Here's how the part is built. I have some questions about the finished solid (model axes, mm). Give positions to 0.01 mm unless a question says otherwise; leave off trailing zeros. Order: outer loops, then holes, each group sorted by start corner. A loop starts at its lowest first (then second) coordinate and runs counter-clockwise, first axis right, second up. Notation, with made-up numbers: (51, -31) -> (107, -31) arc R7 ccw to (107, -25) -> close; hole circle Ø4 at (-39.5, -5). An arc over 180 degrees is marked (long way). Write each question's results on one line, items separated by ' | '. Start each with the question number.
Q1. Imagine slicing it at A-A, the plane z = 4.25. Please give me the cut outline in (x, y).
Q2. Thinking about a two-plate mould opening in X: for faces 1 (the face through (-0.816, -34.994, 3.944)), 2 (the face through (0, -40, 10)), 3 (the face through (-1.24, -30.58, 4.93)), which applies, pulls with the +X half, pulls with the -X half, needs draft (parallel to the pull), parting line crosses it, or undercut?
Q3. Imagine slicing it at C-C, the plane z = 8.5. Please give me the cut outline in (x, y), then the cut area to 3 significant figures.
Q4. I'm going to push flat-ended pins straight in: pin 1 (3 mm diameter, centred on x = -5.12, y = -43.58, fed in from +Z); pin 2 (3 mm diameter, centred on y = -32.5, z = 6, fed in from +X); pin 3 (3 mm diameter, centred on x = 5.66, y = -42.64, fed in from -Z); pin 4 (3 mm diameter, centred on y = -34.5, z = 4, fed in from -X). Where does each tip first touch, or does it pass through?
Q5. Imagine slicing it at B-B, the plane x = -5.25. State how many separate pieces and enclosed holes the cut face has, then the cut area to 3 significant figures.
Q6. I need wall thicknesses on line 1 along Y through (x, z) = (1.5, 9.25); line 2 along Y through (x, z) = (5.5, 9.5); line 3 along Y through (x, z) = (1, 5). Which ranges of each line are inside material? Lowest first, please. Write a range as [from, to].
```python
from build123d import *

# Parameters (mm, degrees)
SKETCH1_R           = 9.5
SKETCH1_R_2         = 1.25
BOSS_EXTRUDE1_DEPTH = 10
CHAMFER1_SIZE       = 2
CHAMFER2_SIZE       = 2


with BuildPart() as part:
    # Sketch1 → Boss-Extrude1 (new body)
    with BuildSketch(Plane.XY):
        with Locations((0, -40)):
            Circle(SKETCH1_R)
        with Locations((5.119700277, -36.415147273)):
            Circle(SKETCH1_R_2, mode=Mode.SUBTRACT)
        with Locations((0.544723392, -46.226216863)):
            Circle(SKETCH1_R_2, mode=Mode.SUBTRACT)
        with Locations((-5.664423669, -37.358635864)):
            Circle(SKETCH1_R_2, mode=Mode.SUBTRACT)
        with Locations((-5.119700277, -43.584852727)):
            Circle(SKETCH1_R_2, mode=Mode.SUBTRACT)
        with Locations((-0.544723392, -33.773783137)):
            Circle(SKETCH1_R_2, mode=Mode.SUBTRACT)
        with Locations((5.664423669, -42.641364136)):
            Circle(SKETCH1_R_2, mode=Mode.SUBTRACT)
    extrude(amount=BOSS_EXTRUDE1_DEPTH)

    # Chamfer1
    chamfer1_edges = [part.edges().sort_by_distance(p)[0] for p in [
        (-6.369700277, -43.584852727, 10),
        (-1.794723392, -33.773783137, 10),
        (4.414423669, -42.641364136, 10),
    ]]
    chamfer(chamfer1_edges, length=CHAMFER1_SIZE - 0.0001)  # a hair under: the kernel refuses the full size

    # Chamfer2
    chamfer2_edges = [part.edges().sort_by_distance(p)[0] for p in [
        (-6.914423669, -37.358635864, 0),
        (3.869700277, -36.415147273, 0),
        (-0.705276608, -46.226216863, 0),
    ]]
    chamfer(chamfer2_edges, length=CHAMFER2_SIZE - 0.0001)  # a hair under: the kernel refuses the full size


solid = part.part
```
Geometry check:
1) outline: circle Ø19 at (0, -40); hole circle Ø2.5 at (-5.66, -37.36); hole circle Ø2.5 at (-5.12, -43.58); hole circle Ø2.5 at (-0.54, -33.77); hole circle Ø2.5 at (0.54, -46.23); hole circle Ø2.5 at (5.12, -36.42); hole circle Ø2.5 at (5.66, -42.64)
2) face 1: undercut | face 2: needs draft | face 3: parting line crosses it
3) outline: circle Ø19 at (0, -40); hole circle Ø2.5 at (-5.66, -37.36); hole circle Ø3.5 at (-5.12, -43.58); hole circle Ø3.5 at (-0.54, -33.77); hole circle Ø2.5 at (0.54, -46.23); hole circle Ø2.5 at (5.12, -36.42); hole circle Ø3.5 at (5.66, -42.64) | area: 240 mm²
4) pin 1: z = 8.25 | pin 2: x = 7.37 | pin 3: z = 0 | pin 4: x = -8.62
5) separate pieces: 3 | enclosed holes: 0 | area: 102 mm²
6) line 1: [-49.38, -47.03], [-45.42, -35.21], [-32.34, -30.62] | line 2: [-47.75, -45.39], [-39.9, -37.61], [-35.22, -32.25] | line 3: [-49.45, -47.39], [-45.06, -30.55]
